from build123d import *

# Parameters (mm, degrees)
SKETCH_1_W          = 90
SKETCH_1_H          = 174
EXTRUDE_1_DEPTH     = 40
SKETCH_2_W          = 40
SKETCH_2_H          = 40
EXTRUDE_2_DEPTH     = 40
SKETCH_3_R          = 7.5
CUT_EXTRUDE_1_DEPTH = 40


with BuildPart() as part:
    # 草图1 → 凸台-拉伸1 (new body)
    with BuildSketch(Plane.XY):
        Rectangle(SKETCH_1_W, SKETCH_1_H)
    extrude(amount=EXTRUDE_1_DEPTH)

    # 草图2 → 凸台-拉伸2 (add)
    with BuildSketch(Plane.XY.offset(40)):
        Rectangle(SKETCH_2_W, SKETCH_2_H)
    extrude(amount=EXTRUDE_2_DEPTH)

    # 草图3 → 切除-拉伸1 (cut)
    with BuildSketch(Plane.XY.offset(80)):
        Circle(SKETCH_3_R)
    extrude(amount=-CUT_EXTRUDE_1_DEPTH, mode=Mode.SUBTRACT)


solid = part.part
Build history of the part. All positions in model axes, mm. A direction names the side the tool comes from. Coordinates: 2 decimals unless noted, no trailing zeros. Order: outer loops, then holes, each group sorted by start corner. A loop starts at its lowest first (then second) coordinate and runs counter-clockwise, first axis right, second up. Notation, with made-up numbers: (-34, 67) - (4, 67) arc R18 cw to (4, 83) - close; hole circle Ø9 at (7.25, 19). An arc over 180 degrees is marked (long way). Write item = value, one per line. Start each with the question number.
1) Saw through at D-D on y = -71. Write the cut outline in (x, z), then the cut area to 3 significant figures.
2) Saw through at A-A on y = -11. Write the cut outline in (x, z).
3) Flat gauge pins, fed straight in: pin 1 Ø1 at (x, z) = (13, 41) entering from +Y; pin 2 Ø8 at (y, z) = (3, 71) entering from -X; pin 3 Ø20 at (y, z) = (4.5, 67) entering from +X. Where does each tip first touch, or does it go through?
4) 3-axis set-ups, long thin cutter, end or side, ignore diameter. For faces 5 (the face through (-7.493, 0.33, 60.28)), 6 (the face through (0, 20, 60)), 7 (the face through (-1, 1, 0)), 8 (the face through (20, 0, 60)): which of +Z, -Z, +X, -X, +Y, -Y reach the whole face in a straight line?
5) Wall check: line 1 along Y through (x, z) = (0, 69); line 2 along Z through (x, y) = (-22.5, -43.5); line 3 along X through (y, z) = (2, 56). Give the ranges that are in metal, low to high. Write a range as from..to.
6) Saw through at C-C on x = 0. Write the cut outline in (y, z).
7) Two-plate mould, pull along X, no slides. Class faces 1 (the face through (45, -1, 20)), 2 (the face through (0, 0, 40)), 3 (the face through (-20, 0, 60)), 4 (the face through (0, -20, 60)): pulls with the +X half, pulls with the -X half, needs draft (parallel to the pull), parting line crosses it, or undercut.
8) Saw through at B-B on x = -9.5. Write the cut outline in (y, z).
From the geometry:
q1.outline = (-45, 0) - (45, 0) - (45, 40) - (-45, 40) - close
q1.area = 3,600 mm^2
q2.outline = (-45, 0) - (45, 0) - (45, 40) - (20, 40) - (20, 80) - (-20, 80) - (-20, 40) - (-45, 40) - close
q3.pin_1 = 20
q3.pin_2 = -20
q3.pin_3 = 20
q4.face_5 = +Z
q4.face_6 = +Z, +X, -X, +Y
q4.face_7 = -Z, +X, -X, +Y, -Y
q4.face_8 = +Z, +X, +Y, -Y
q5.line_1 = -20..-7.5, 7.5..20
q5.line_2 = 0..40
q5.line_3 = -20..-7.23, 7.23..20
q6.outline = (-87, 0) - (87, 0) - (87, 40) - (20, 40) - (20, 80) - (7.5, 80) - (7.5, 40) - (-7.5, 40) - (-7.5, 80) - (-20, 80) - (-20, 40) - (-87, 40) - close
q7.face_1 = pulls with the +X half
q7.face_2 = undercut
q7.face_3 = pulls with the -X half
q7.face_4 = needs draft
q8.outline = (-87, 0) - (87, 0) - (87, 40) - (20, 40) - (20, 80) - (-20, 80) - (-20, 40) - (-87, 40) - close
